Verification items for the finished model (mm, model axes). Face numbers are marked on the shaded views. A direction names the side the tool comes from. Give positions to 0.01 mm unless a question says otherwise; leave off trailing zeros. Order: outer loops, then holes, each group sorted by start corner. A loop starts at its lowest first (then second) coordinate and runs counter-clockwise, first axis right, second up. Notation, with made-up numbers: M 56.5,-35 L 76.5,-35 A20 cw 76.5,-28 Z; hole C 29.5,71 d7. An arc over 180 degrees is marked long. Answer as a JSON object with one key per item and string values.
```python
from build123d import *

# Parameters (mm, degrees)
BOSS_EXTRUDE1_DEPTH     = 23
SKETCH3_W               = 22
SKETCH3_H               = 74
BOSS_EXTRUDE2_DEPTH     = 1.5
FILLET1_R               = 8
CUT_EXTRUDE1_DEPTH      = 50.53029376
CUT_EXTRUDE1_DEPTH_BACK = 50.53029376
SKETCH4_R               = 0.75


with BuildPart() as part:
    # Sketch2 → Boss-Extrude1 (new body)
    with BuildSketch(Plane(origin=(0, 0, 0), x_dir=(1, 0, 0), z_dir=(0, 1, 0))):
        Polygon((-10.5, -35.5), (10, -35.5), (10, -37), (-12, -37), (-12, 37), (10, 37), (10, 35.5), (-10.5, 35.5), align=None)
    extrude(amount=BOSS_EXTRUDE1_DEPTH)

    # Sketch3 → Boss-Extrude2 (add)
    with BuildSketch(Plane(origin=(0, 23, 0), x_dir=(1, 0, 0), z_dir=(0, 1, 0))):
        with Locations((-1, 0)):
            Rectangle(SKETCH3_W, SKETCH3_H)
    extrude(amount=BOSS_EXTRUDE2_DEPTH)

    # Fillet1
    fillet1_edges = [part.edges().sort_by_distance(p)[0] for p in [
        (-12, 24.5, 0),
        (-10.5, 23, 0),
    ]]
    fillet(fillet1_edges, radius=FILLET1_R)

    # Sketch4 → Cut-Extrude1 (cut, two sides: drawn at the far end of the back side and taken through both)
    with BuildSketch(Plane.ZY.offset(12).offset(-CUT_EXTRUDE1_DEPTH_BACK)):
        with Locations((-25, 1.5)):
            Circle(SKETCH4_R)
        with Locations((0, 1.5)):
            Circle(SKETCH4_R)
        with Locations((25, 1.5)):
            Circle(SKETCH4_R)
    extrude(amount=CUT_EXTRUDE1_DEPTH + CUT_EXTRUDE1_DEPTH_BACK, mode=Mode.SUBTRACT)


solid = part.part
```
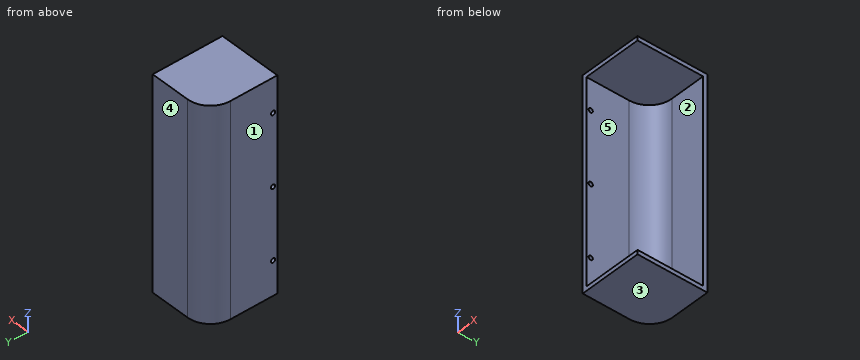
Q1. Gauge pin test, flat ends, axial feed: pin 1 Ø1.4 at (y, z) = (1.5, 25) entering from +X; pin 2 Ø2.5 at (y, z) = (1.5, 0) entering from -X; pin 3 Ø4 at (x, z) = (3, -7) entering from -Y; pin 4 Ø5 at (y, z) = (6, -8) entering from +X. Record the tip position at first contact, or that the pin passes through.
Resolved:
{"pin 1": "passes through", "pin 2": "stops at x = -12", "pin 3": "stops at y = 23", "pin 4": "stops at x = -10.5"}
Q2. Section check C-C on y = 10. Record the cut outline in (x, z).
Resolved:
{"outline": "M -12,-37 L 10,-37 L 10,-35.5 L -10.5,-35.5 L -10.5,35.5 L 10,35.5 L 10,37 L -12,37 Z"}
Q3. Section check D-D on x = 4.25. Record the cut outline in (y, z).
Resolved:
{"outline": "M 0,-37 L 24.5,-37 L 24.5,37 L 0,37 L 0,35.5 L 23,35.5 L 23,-35.5 L 0,-35.5 Z"}
Q4. Tool access check on the marked faces 1 and 2. Record the directions out of +Z, -Z, +X, -X, +Y, -Y that give a thin tool (end or side, any length) a straight path to the whole face; none if there is none.
Resolved:
{"face 1": "+Z, -Z, -X, +Y, -Y", "face 2": "+X, -Y"}
Q5. Release check for a two-part mould opening along Z. For the marked faces 3, 4 and 5 record: +Z half, -Z half, draft (parallel to the pull), parting line (faces both ways), or undercut.
Resolved:
{"face 3": "-Z half", "face 4": "draft", "face 5": "undercut"}
Q6. Section check B-B on z = -25. Record the cut outline in (x, y), then the cut area to 4 significant figures.
Resolved:
{"outline": "M -12,0 L -10.5,0 L -10.5,0.75 L -12,0.75 Z; M -12,2.25 L -10.5,2.25 L -10.5,15 A8 cw -2.5,23 L 10,23 L 10,24.5 L -4,24.5 A8 ccw -12,16.5 Z", "area": "65.25 mm²"}
Q7. Material ranges on L1, parallel to Z at x = -11.4, y = 1.5; L2, parallel to Z at x = 3.25, y = 8; L3, parallel to Y at x = 5.75, z = 27.5, recorded low to high.
Resolved:
{"L1": "z = -37 to -25.75, -24.25 to -0.75, 0.75 to 24.25, 25.75 to 37", "L2": "z = -37 to -35.5, 35.5 to 37", "L3": "y = 23 to 24.5"}
Q8. Section check A-A on y = 1.5. Record the cut outline in (x, z), then the cut area to 3 significant figures.
Resolved:
{"outline": "M -12,-37 L 10,-37 L 10,-35.5 L -10.5,-35.5 L -10.5,-25.75 L -12,-25.75 Z; M -12,-24.25 L -10.5,-24.25 L -10.5,-0.75 L -12,-0.75 Z; M -12,0.75 L -10.5,0.75 L -10.5,24.25 L -12,24.25 Z; M -12,25.75 L -10.5,25.75 L -10.5,35.5 L 10,35.5 L 10,37 L -12,37 Z", "area": "166 mm²"}
